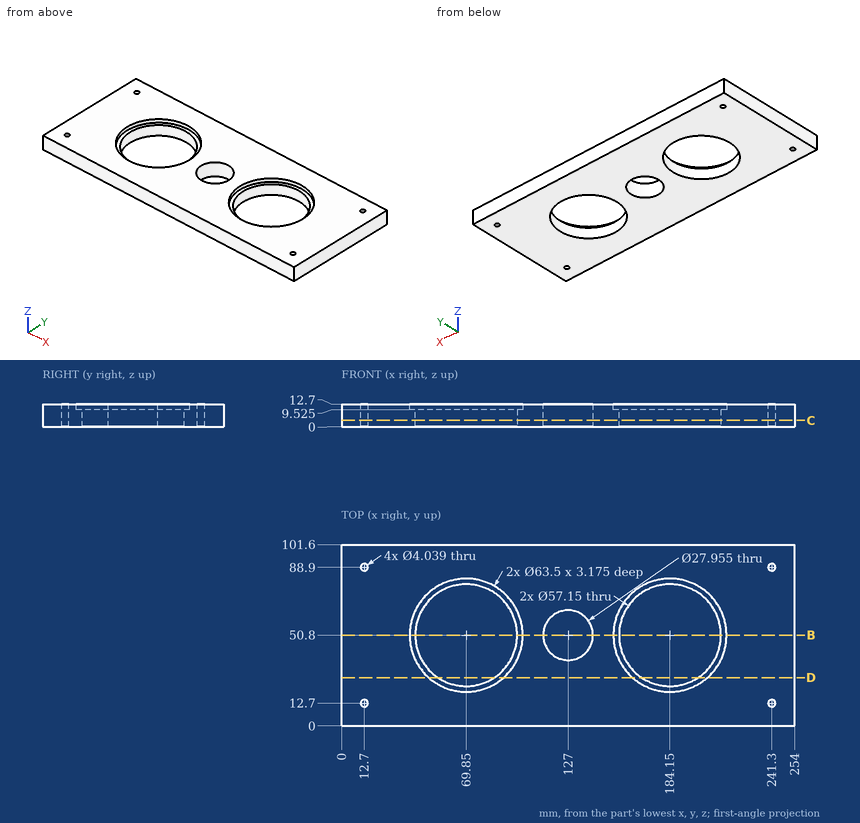
Job drawing, mm, ordinate dimensions from the low corner. One solid piece. Coordinates: 2 decimals unless noted, no trailing zeros. Write each loop counter-clockwise with the first axis right and the second up, starting at its lowest first coordinate (ties: lowest second). Pieces come first, ordered by that corner, then holes. Notation, with made-up numbers: (-6, 69) -> (53, 69) arc R13 ccw to (53, 75) -> close; hole circle Ø8 at (-37, -19.75). An arc over 180 degrees is marked (long way). Use CSV: the item, a comma, the result in double quotes. Start each with the question number.
Item 1: Band-saw the part on C-C, the plane z = 3.5. Give the number of separate pieces and of enclosed holes in the cut face, plus the area to 3 significant figures.
Item 2: Band-saw the part on B-B, the plane y = 50.8. Write the cut outline in (x, z) (1 decimal).
Item 3: Wall check: probe 1 along Y at (x, z) = (12.7, 7.75); probe 2 along X at (y, z) = (88.9, 9.5); probe 3 along X at (y, z) = (32, 6). Give the ranges that are in metal, low to high.
Item 4: Drop flat-ended pins along their axis: P1, Ø3, axis at y = 11.5, z = 10, coming from the -X side; P2, Ø3.5, axis at x = 241.3, y = 12.7, coming from the +Z side. Give the stop position or say it passes through.
Item 5: Band-saw the part on D-D, the plane y = 27. Write the cut outline in (x, z) (1 decimal), plus the area to 3 significant figures.
Response values:
1,separate pieces,"1"
1,enclosed holes,"7"
1,area,"20,000 mm2"
2,outline,"(0, 0) -> (41.3, 0) -> (41.3, 9.5) -> (38.1, 9.5) -> (38.1, 12.7) -> (0, 12.7) -> close; (98.4, 0) -> (113, 0) -> (113, 12.7) -> (101.6, 12.7) -> (101.6, 9.5) -> (98.4, 9.5) -> close; (141, 0) -> (155.6, 0) -> (155.6, 9.5) -> (152.4, 9.5) -> (152.4, 12.7) -> (141, 12.7) -> close; (212.7, 0) -> (254, 0) -> (254, 12.7) -> (215.9, 12.7) -> (215.9, 9.5) -> (212.7, 9.5) -> close"
3,probe 1,"y = 0 to 10.68, 14.72 to 86.88, 90.92 to 101.6"
3,probe 2,"x = 0 to 10.68, 14.72 to 239.28, 243.32 to 254"
3,probe 3,"x = 0 to 48.33, 91.37 to 162.63, 205.67 to 254"
4,P1,"stops at x = 0"
4,P2,"passes through"
5,outline,"(0, 0) -> (54, 0) -> (54, 9.5) -> (48.8, 9.5) -> (48.8, 12.7) -> (0, 12.7) -> close; (85.7, 0) -> (168.3, 0) -> (168.3, 9.5) -> (163.1, 9.5) -> (163.1, 12.7) -> (90.9, 12.7) -> (90.9, 9.5) -> (85.7, 9.5) -> close; (200, 0) -> (254, 0) -> (254, 12.7) -> (205.2, 12.7) -> (205.2, 9.5) -> (200, 9.5) -> close"
5,area,"2,360 mm2"
